from build123d import *

# Parameters (mm, degrees)
F0_W     = 12
F0_H     = 12
F1_DEPTH = 10
F2_DEPTH = 9
F3_R     = 2
F4_DEPTH = 13
F5_R     = 7
F6_R     = 5


with BuildPart() as f1:
    # F0 (on Front) → F1 (new body)
    with BuildSketch(Plane.XZ):
        Rectangle(F0_W, F0_H)
    extrude(amount=F1_DEPTH)

    # F2 (add): a face of the model
    f2_faces = [f1.faces().sort_by_distance(p)[0] for p in [
        (0, 0, 0),
    ]]
    extrude(f2_faces, amount=F2_DEPTH)

    # F3 (on face) → F4 (cut)
    with BuildSketch(Plane.XY.offset(6)):
        with Locations((0, 4.5)):
            Circle(F3_R)
    extrude(amount=-F4_DEPTH, mode=Mode.SUBTRACT)

    # F5
    f5_edges = [f1.edges().sort_by_distance(p)[0] for p in [
        (6, 9, 0),
    ]]
    fillet(f5_edges, radius=F5_R)

    # F6
    f6_edges = [f1.edges().sort_by_distance(p)[0] for p in [
        (6, -10, 0),
        (-6, -10, 0),
    ]]
    fillet(f6_edges, radius=F6_R)


solid = f1.part
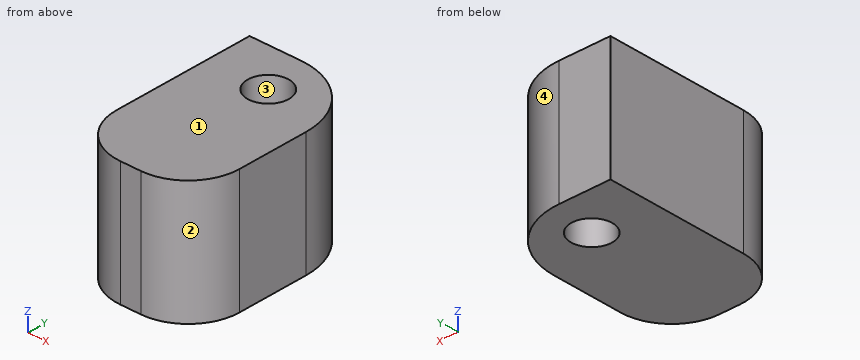
The model under review builds one solid part; all positions refer to its coordinate system, in mm. Face numbers are marked on the shaded views. Round coordinates to 2 decimals unless told otherwise and drop trailing zeros. Order: outer loops, then holes, each group sorted by start corner. A loop starts at its lowest first (then second) coordinate and runs counter-clockwise, first axis right, second up. Notation, with made-up numbers: (33, 74) -> (87, 74) arc R29 cw to (87, 108) -> close; hole circle Ø6 at (15.5, 29.5). An arc over 180 degrees is marked (long way). Write item = value, one per line. Start each with the question number.
Item 1: Consider section D-D on x = -4. Write out the cut boundary in (y, z), plus the area to 3 significant figures.
Item 2: Consider section C-C on y = 4.5. Write out the cut boundary in (x, z), plus the area to 3 significant figures.
Item 3: Consider section B-B on x = 0. Write out the cut boundary in (y, z), plus the area to 3 significant figures.
Item 4: Clearance check with flat-ended pins moving along their axes: pin 1 Ø6 at (x, z) = (2, 3.5) entering from +Y; pin 2 Ø4 at (x, z) = (-3.5, -4.5) entering from -Y. State where each tip first meets the part, or that it passes through.
Item 5: Mouldability with a two-part tool opening along Y and no side actions: class the marked faces 1, 2, 3 and 4 as released by +Y, released by -Y, zero draft, split by the parting line, or undercut.
Item 6: Consider section A-A on z = 3. Write out the cut boundary in (x, y), plus the area to 3 significant figures.
Item 7: For line 1 along Y through (x, z) = (0, -1.5); line 2 along Y through (x, z) = (1.5, -4.5); line 3 along X through (y, z) = (-7.5, 5), list the stretches that pass through material, from the lowest coordinate up.
Conclusion:
q1.outline = (-9, -6) -> (9, -6) -> (9, 6) -> (-9, 6) -> close
q1.area = 216 mm2
q2.outline = (-6, -6) -> (-2, -6) -> (-2, 6) -> (-6, 6) -> close; (2, -6) -> (5.54, -6) -> (5.54, 6) -> (2, 6) -> close
q2.area = 90.5 mm2
q3.outline = (-10, -6) -> (2.5, -6) -> (2.5, 6) -> (-10, 6) -> close; (6.5, -6) -> (8.93, -6) -> (8.93, 6) -> (6.5, 6) -> close
q3.area = 179 mm2
q4.pin_1 = 9
q4.pin_2 = -9.97
q5.face_1 = zero draft
q5.face_2 = released by -Y
q5.face_3 = undercut
q5.face_4 = released by +Y
q6.outline = (-6, -5) arc R5 ccw to (-1, -10) -> (1, -10) arc R5 ccw to (6, -5) -> (6, 2) arc R7 ccw to (-1, 9) -> (-6, 9) -> close; hole circle Ø4 at (0, 4.5)
q6.area = 194 mm2
q7.line_1 = -10 to 2.5, 6.5 to 8.93
q7.line_2 = -9.97 to 3.18, 5.82 to 8.54
q7.line_3 = -5.33 to 5.33
